Autodesk Fusion 360 part; units mm, degrees
sketch "Sketch1" plane through (0, 0, 0) normal (0, 0, 1) x (1, 0, 0)
  line L0 (-60, 70) -> (40, 70)
  line L1 (40, 70) -> (40, 10)
  line L2 (40, 10) -> (-60, 10)
  line L3 (-60, 10) -> (-60, 70)
  line L4 (-60, 70) -> (40, 70)
  line L5 (40, 70) -> (40, 50)
  line L6 (40, 50) -> (-60, 50)
  line L7 (-60, 50) -> (-60, 70)
  line L8 (-60, 70) -> (-35, 70)
  line L9 (-35, 70) -> (15, 70)
  line L10 (15, 70) -> (15, 50)
  line L11 (15, 50) -> (-35, 50)
  line L12 (-35, 50) -> (-35, 70)
  dimension "d1" = 100
  dimension "d2" = 60
extrude "Extrude1" add sketch "Sketch1" along normal blind 20 contours L1 L2 L3 L6 L11
extrude "Extrude2" add sketch "Sketch1" along normal blind 45 contours L0 L3 L4 L6 L7 L8 L12
extrude "Extrude3" add sketch "Sketch1" along normal blind 45 contours L0 L1 L4 L5 L6 L10
extrude "Extrude4" add sketch "Sketch1" along normal blind 45 contours L0 L4 L6 L9 L10 L11 L12
sketch "Sketch2" plane through (0, 50, 0) normal (0, -1, 0) x (1, 0, 0)
  line L0 (-60, 20) -> (40, 20)
  line L1 (40, 20) -> (40, 45)
  line L2 (40, 45) -> (-60, 45)
  line L3 (-60, 45) -> (-60, 20)
sketch "Sketch3" plane through (0, 50, 0) normal (0, -1, 0) x (1, 0, 0)
  line L0 (-35, 45) -> (-30, 45)
  circle A0 centre (-10, 45) radius 20
  line L1 (10, 45) -> (15, 45)
  arc A1 (15, 45) -> (-35, 45) centre (-10, 45) ccw
  dimension "d12" = 40
  dimension "d13" = 50
hole "Hole1" at (-10, 50, 45) direction (0, 1, 0) diameter 40 depth 600 tip angle 118
extrude "Extrude5" add sketch "Sketch3" against normal blind 20 contours L0 A0 L1 A1
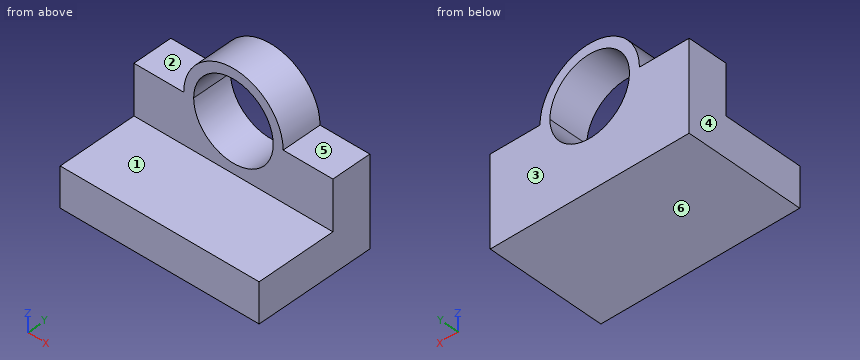
Model file for the job. Use its own axes, mm. Face numbers are marked on the shaded views. A direction names the side the tool comes from. Round coordinates to 2 decimals unless told otherwise and drop trailing zeros. Loops run counter-clockwise (first coordinate to the right, second up) from the corner with the lowest first, then second, coordinate; pieces in that order, holes last. Notation, with made-up numbers: (38.25, 64.5) -> (95.25, 64.5) arc R23 ccw to (95.25, 91.5) -> close; hole circle Ø11 at (3.5, -0.5). An arc over 180 degrees is marked (long way). Answer as CSV lines item,"result". Start each with the question number.
1) Tool access for the marked faces 1, 2 and 3: list every direction of +Z, -Z, +X, -X, +Y, -Y with a clear straight run to the whole face (end or side of a thin tool).
2) Slice it at A-A (x = -10). List the corners of the cut face in (y, z), plus the area to 3 significant figures.
3) Probe line 1 along Z through (x, y) = (33.5, 29); line 2 along X through (y, z) = (55, 44.5); line 3 along Z through (x, y) = (-28, 55). List the from-to ranges inside material, lowest first.
4) Slice it at D-D (z = 57). List the corners of the cut face in (x, y).
5) Mould opens along Z. For the marked faces 4, 5 and 6 say: +Z half, -Z half, draft (parallel to the pull), parting line (faces both ways), or undercut.
6) Slice it at B-B (z = 37). List the corners of the cut face in (x, y), plus the area to 3 significant figures.
7) Pin check, flat tips, straight feed: P1, Ø16, axis at x = -51, y = 56, coming from the +Z side; P2, Ø10, axis at x = -29.5, y = 19, coming from the +Z side. Stop position of each tip, or through.
8) Slice it at C-C (x = 22). List the corners of the cut face in (y, z).
Filled in:
1,face 1,"+Z, +X, -X, -Y"
1,face 2,"+Z, -X, +Y, -Y"
1,face 3,"+Z, -Z, +X, -X, +Y"
2,outline,"(10, 0) -> (70, 0) -> (70, 25) -> (50, 25) -> (50, 20) -> (10, 20) -> close; (50, 65) -> (70, 65) -> (70, 70) -> (50, 70) -> close"
2,area,"1,400 mm2"
3,line 1,"z = 0 to 20"
3,line 2,"x = -60 to -29.99, 9.99 to 40"
3,line 3,"z = 0 to 36.28, 53.72 to 62.35"
4,outline,"(-31.93, 50) -> (-26, 50) -> (-26, 70) -> (-31.93, 70) -> close; (6, 50) -> (11.93, 50) -> (11.93, 70) -> (6, 70) -> close"
5,face 4,"draft"
5,face 5,"+Z half"
5,face 6,"-Z half"
6,outline,"(-60, 50) -> (-28.33, 50) -> (-28.33, 70) -> (-60, 70) -> close; (8.33, 50) -> (40, 50) -> (40, 70) -> (8.33, 70) -> close"
6,area,"1,270 mm2"
7,P1,"stops at z = 45"
7,P2,"stops at z = 20"
8,outline,"(10, 0) -> (70, 0) -> (70, 45) -> (50, 45) -> (50, 20) -> (10, 20) -> close"
